Autodesk Inventor part; units mm, degrees
ref_plane "YZ Plane" through (0, 0, 0) normal (1, 0, 0) x (0, 1, 0)
ref_plane "XZ Plane" through (0, 0, 0) normal (0, 1, 0) x (-1, 0, 0)
ref_plane "XY Plane" through (0, 0, 0) normal (0, 0, 1) x (1, 0, 0)
sketch "Sketch1" plane through (0, 0, 0) normal (0, 0, 1) x (1, 0, 0)
  line L0 (-42.5, 28) -> (42.5, 28)
  line L1 (42.5, 28) -> (42.5, -28)
  line L2 (42.5, -28) -> (-42.5, -28)
  line L3 (-42.5, -28) -> (-42.5, 28)
  point P0 (0, 0)
  point P1 (0, 28)
  point P2 (-42.5, 0)
  dimension "d0" = 85
  dimension "d1" = 56
extrude "Extrusion1" add sketch "Sketch1" along normal blind 2
fillet "Fillet1" radius 3 4 edges at (42.5, 28, 1) (42.5, -28, 1) (-42.5, -28, 1) (-42.5, 28, 1)
sketch "Sketch2" plane through (0, 0, 2) normal (0, 0, 1) x (1, 0, 0)
  line L0 (39.5, 28) -> (-39.5, 28)
  line L1 (-42.5, 25) -> (-42.5, -25)
  line L2 (-39.5, -28) -> (39.5, -28)
  point P0 (0, 0)
  point P1 (-39, 24.5)
  point P2 (19, 24.5)
  point P3 (-39, -24.5)
  point P4 (19, -24.5)
  dimension "d5" = 3.5
  dimension "d6" = 3.5
  dimension "d7" = 58
  dimension "d8" = 3.5
hole "Hole1" at (-39, 24.5, 2) at (19, 24.5, 2) at (-39, -24.5, 2) at (19, -24.5, 2) direction (0, 0, -1) diameter 2.7 end through all
sketch "Sketch3" plane through (0, 0, 2) normal (0, 0, 1) x (1, 0, 0)
  line L0 (-66.5402, 48.8384) -> (82.1472, 48.8384) construction
  line L1 (82.1472, 48.8384) -> (82.1472, -46.7464) construction
  line L2 (82.1472, -46.7464) -> (-66.5402, -46.7464) construction
  line L3 (-66.5402, -46.7464) -> (-66.5402, 48.8384) construction
  line L4 (27.7, -12.375) -> (45.3, -12.375)
  line L5 (45.3, -12.375) -> (45.3, -25.625)
  line L6 (45.3, -25.625) -> (27.7, -25.625)
  line L7 (27.7, -25.625) -> (27.7, -12.375)
  line L8 (27.7, 5.5) -> (45.3, 5.5)
  line L9 (45.3, 5.5) -> (45.3, -7.5)
  line L10 (45.3, -7.5) -> (27.7, -7.5)
  line L11 (27.7, -7.5) -> (27.7, 5.5)
  line L12 (23.9, 25.5) -> (45.3, 25.5)
  line L13 (45.3, 25.5) -> (45.3, 10)
  line L14 (45.3, 10) -> (23.9, 10)
  line L15 (23.9, 10) -> (23.9, 25.5)
  line L16 (-20.9, 12) -> (-5.9, 12)
  line L17 (-5.9, 12) -> (-5.9, -3)
  line L18 (-5.9, -3) -> (-20.9, -3)
  line L19 (-20.9, -3) -> (-20.9, 12)
  line L20 (-35.75, -21.75) -> (-27, -21.75)
  line L21 (-27, -21.75) -> (-27, -29)
  line L22 (-27, -29) -> (-35.75, -29)
  line L23 (-35.75, -29) -> (-35.75, -21.75)
  line L24 (-13.5, -21.25) -> (-19.75, -21.25)
  line L25 (-19.75, -21.25) -> (-19.75, -29.25)
  line L26 (-19.75, -29.25) -> (-13.5, -29.25)
  line L27 (-13.5, -29.25) -> (-13.5, -21.25)
  line L28 (-6.25, -21.25) -> (0, -21.25)
  line L29 (0, -21.25) -> (0, -29.25)
  line L30 (0, -29.25) -> (-6.25, -29.25)
  line L31 (-6.25, -29.25) -> (-6.25, -21.25)
  line L32 (7.75, -15.25) -> (14.75, -15.25)
  line L33 (14.75, -15.25) -> (14.75, -30.25)
  line L34 (14.75, -30.25) -> (7.75, -30.25)
  line L35 (7.75, -30.25) -> (7.75, -15.25)
  line L36 (2.5, -5) -> (6.5, -5)
  line L37 (6.5, -5) -> (6.5, -27.5)
  line L38 (6.5, -27.5) -> (2.5, -27.5)
  line L39 (2.5, -27.5) -> (2.5, -5)
  line L40 (-37.25, -11) -> (-41.25, -11)
  line L41 (-41.25, -11) -> (-41.25, 11.25)
  line L42 (-41.25, 11.25) -> (-37.25, 11.25)
  line L43 (-37.25, 11.25) -> (-37.25, -11)
  line L44 (-35.5, 27) -> (15.25, 27)
  line L45 (15.25, 27) -> (15.25, 22)
  line L46 (15.25, 22) -> (-35.5, 22)
  line L47 (-35.5, 22) -> (-35.5, 27)
  line L48 (-42.5, 25) -> (-42.5, -25)
  line L49 (39.5, 28) -> (-39.5, 28)
  line L50 (-39.5, -28) -> (39.5, -28)
  line L51 (42.5, -25) -> (42.5, 25)
  point P0 (0, 0)
  point P1 (-39.25, 11.25)
  point P2 (45.3, -19)
  point P3 (45.3, -1)
  point P4 (45.3, 17.75)
  dimension "d55" = 7
  dimension "d56" = 50.75
  dimension "d57" = 5
  dimension "d58" = 1
  dimension "d59" = 16.75
  dimension "d60" = 22.25
  dimension "d61" = 4
  dimension "d62" = 1.25
  dimension "d63" = 1
  dimension "d64" = 1.25
  dimension "d65" = 7.25
  dimension "d66" = 8.75
  dimension "d67" = 6.75
  dimension "d68" = 22.75
  dimension "d69" = 6.25
  dimension "d70" = 6.75
  dimension "d71" = 36.25
  dimension "d72" = 6.25
  dimension "d73" = 4
  dimension "d74" = 22.5
  dimension "d75" = 45
  dimension "d76" = 0.5
  dimension "d77" = 7
  dimension "d78" = 2.25
  dimension "d79" = 27.75
  dimension "d80" = 15
  dimension "d81" = 9
  dimension "d82" = 17.6
  dimension "d83" = 13.25
  dimension "d84" = 2.8
  dimension "d85" = 13
  dimension "d86" = 27
  dimension "d87" = 21.4
  dimension "d88" = 15.5
  dimension "d89" = 45.75
  dimension "d90" = 15
  dimension "d91" = 15
  dimension "d92" = 16
  dimension "d93" = 21.6
extrude "Extrusion2" add sketch "Sketch3" along normal blind 5.5 contours L40 L41 L42 L43
extrude "Extrusion3" add sketch "Sketch3" along normal blind 8.5 contours L44 L45 L46 L47
extrude "Extrusion4" add sketch "Sketch3" along normal blind 2.4 contours L16 L17 L18 L19
extrude "Extrusion5" add sketch "Sketch3" along normal blind 3.2 contours L20 L21 L50 L23 | L50 L21 L22 L23
extrude "Extrusion6" add sketch "Sketch3" along normal blind 3 contours L25 L24 L27 L50 | L50 L27 L26 L25
extrude "Extrusion7" add sketch "Sketch3" along normal blind 3 contours L31 L28 L29 L50 | L50 L29 L30 L31
extrude "Extrusion8" add sketch "Sketch3" along normal blind 5.5 contours L36 L37 L38 L39
extrude "Extrusion9" add sketch "Sketch3" along normal blind 6 contours L35 L32 L33 L50 | L50 L33 L34 L35
extrude "Extrusion10" add sketch "Sketch3" along normal blind 16 contours L4 L5 L6 L7
extrude "Extrusion11" add sketch "Sketch3" along normal blind 16 contours L10 L11 L8 L51 | L51 L8 L9 L10
extrude "Extrusion12" add sketch "Sketch3" along normal blind 13.5 contours L14 L15 L12 L13
sketch "Sketch4" plane through (0, 0, 4.4) normal (0, 0, 1) x (1, 0, 0)
  line L0 (-5.9, -3) -> (-5.9, 12)
  line L1 (-20.9, 12) -> (-5.9, 12)
  line L2 (-5.9, -3) -> (-20.9, -3)
  line L3 (-20.9, -3) -> (-20.9, 12)
  line L4 (-20.9, 12) -> (-5.9, 12)
  line L5 (-5.9, 12) -> (-5.9, -3)
  point P0 (0, 0)
extrude "Extrusion13" cut sketch "Sketch4" against normal blind 2
properties part number "PI 4 B SPACE MODEL"
For this review, take the finished solid that the model builds, in its own axes (mm). A direction names the side the tool comes from. Coordinates: 2 decimals unless noted, no trailing zeros. Loops run counter-clockwise (first coordinate to the right, second up) from the corner with the lowest first, then second, coordinate; pieces in that order, holes last.
1. Mouldability with a two-part tool opening along Y and no side actions: class faces 1 (the flat face through (36, 5.5, 10)), 2 (the flat face through (-39, 11.25, 5)), 3 (the flat face through (0, -25, 3)) as +Y half, -Y half, draft (parallel to the pull), parting line (faces both ways), or undercut.
2. For line 1 (Y direction, x = 19, z = 1); line 2 (X direction, y = 24.5, z = 0.6); line 3 (Z direction, x = 23.5, y = -9.5), list the stretches that pass through material, from the lowest coordinate up.
3. Add section B-B, the plane x = 19. Give the boundary of the cut face in (y, z).
4. For faces 4 (the flat face through (15.25, 25, 6)), 5 (the flat face through (44, -1, 2)), 6 (the flat face through (-41.25, 0, 5)), 7 (the flat face through (4, -16, 7.5)), 8 (the flat face through (-3, -25, 5)), list the 3-axis set-ups (+Z, -Z, +X, -X, +Y, -Y) from which the entire face can be reached by the end or side of a thin tool; tool diameter is ignored.
5. Add section C-C, the plane z = 14.5. Give the boundary of the cut face in (x, y) (3 decimals).
6. Insertion check: P1, Ø1, axis at y = -1.5, z = 12, coming from the -X side; P2, Ø2.5, axis at y = -27, z = 3, coming from the -X side; P3, Ø12, axis at x = -30.5, y = -9, coming from the +Z side; P4, Ø2.5, axis at x = -39, y = -24.5, coming from the +Z side. Each pin has a flat end and moves straight along its axis. Give the tip position at first contact, or say it passes through.
7. Add section D-D, the plane x = -5. Give the boundary of the cut face in (y, z).
8. Add section A-A, the plane z = 6.5. Give the boundary of the cut face in (x, y) (3 decimals), then the cut area to 3 significant figures.
Result:
1. face 1: undercut
1. face 2: +Y half
1. face 3: draft
2. line 1: y = -28 to -25.85, -23.15 to 23.15, 25.85 to 28
2. line 2: x = -42.5 to -40.35, -37.65 to 17.65, 20.35 to 42.5
2. line 3: z = 0 to 2
3. outline: (-28, 0) - (-25.85, 0) - (-25.85, 2) - (-28, 2) - close; (-23.15, 0) - (23.15, 0) - (23.15, 2) - (-23.15, 2) - close; (25.85, 0) - (28, 0) - (28, 2) - (25.85, 2) - close
4. face 4: +Z, +Y, -Y
4. face 5: -Z, +X, +Y, -Y
4. face 6: +Z, -X, +Y, -Y
4. face 7: +Z, -X, -Y
4. face 8: +Z, -Y
5. outline: (23.9, 10) - (45.3, 10) - (45.3, 25.5) - (23.9, 25.5) - close; (27.7, -25.625) - (45.3, -25.625) - (45.3, -12.375) - (27.7, -12.375) - close; (27.7, -7.5) - (45.3, -7.5) - (45.3, 5.5) - (27.7, 5.5) - close
6. P1: stops at x = 27.7
6. P2: stops at x = -42.23
6. P3: stops at z = 2
6. P4: passes through
7. outline: (-29.25, 2) - (-28, 2) - (-28, 0) - (28, 0) - (28, 2) - (27, 2) - (27, 10.5) - (22, 10.5) - (22, 2) - (-21.25, 2) - (-21.25, 5) - (-29.25, 5) - close
8. outline: (-41.25, -11) - (-37.25, -11) - (-37.25, 11.25) - (-41.25, 11.25) - close; (-35.5, 22) - (15.25, 22) - (15.25, 27) - (-35.5, 27) - close; (2.5, -27.5) - (6.5, -27.5) - (6.5, -5) - (2.5, -5) - close; (7.75, -30.25) - (14.75, -30.25) - (14.75, -15.25) - (7.75, -15.25) - close; (23.9, 10) - (45.3, 10) - (45.3, 25.5) - (23.9, 25.5) - close; (27.7, -25.625) - (45.3, -25.625) - (45.3, -12.375) - (27.7, -12.375) - close; (27.7, -7.5) - (45.3, -7.5) - (45.3, 5.5) - (27.7, 5.5) - close
8. area: 1,330 mm2
